Verification items for this drawing (mm, ordinates from the low corner). A direction names the side the tool comes from. Round coordinates to 2 decimals unless told otherwise and drop trailing zeros. Order: outer loops, then holes, each group sorted by start corner. A loop starts at its lowest first (then second) coordinate and runs counter-clockwise, first axis right, second up. Notation, with made-up numbers: M 54,-2 L 67,-2 A22 ccw 67,37 Z; hole C 20.5,-23 d3. An arc over 180 degrees is marked long. One line per item, written item: value. Start each with the question number.
(1) Cross-section at B-B, the plane z = 1.75. Enter the section's corners in (x, y).
(2) Thickness scan on L1, parallel to X at y = 2.25, z = 1.75; L2, parallel to X at y = 3.5, z = 3; L3, parallel to Z at x = 9.25, y = 4.5. Record the ranges inside material, lowest first.
(3) Cross-section at C-C, the plane x = 7.5. Enter the section's corners in (y, z), and give its area (3 significant figures).
(4) Release check for a two-part mould opening along Y. For the marked faces 4, 5 and 6 record: released by +Y, released by -Y, zero draft, split by the parting line, or undercut.
(5) Access from +Z, -Z, +X, -X, +Y, -Y to the whole of each face (thin tool, end or side, straight path). Record for the marked faces 1, 2 and 3.
(6) Cross-section at D-D, the plane z = 3.25. Enter the section's corners in (x, y) (1 decimal).
(7) Cross-section at A-A, the plane y = 3.5. Enter the section's corners in (x, z) (1 decimal).
(8) Depth check by flat-ended pin: pin 1 Ø4 at (x, z) = (11.5, 3.5) entering from -Y; pin 2 Ø1 at (x, z) = (15, 4.5) entering from +Y. Enter the tip coordinate at first touch or a pass-through.
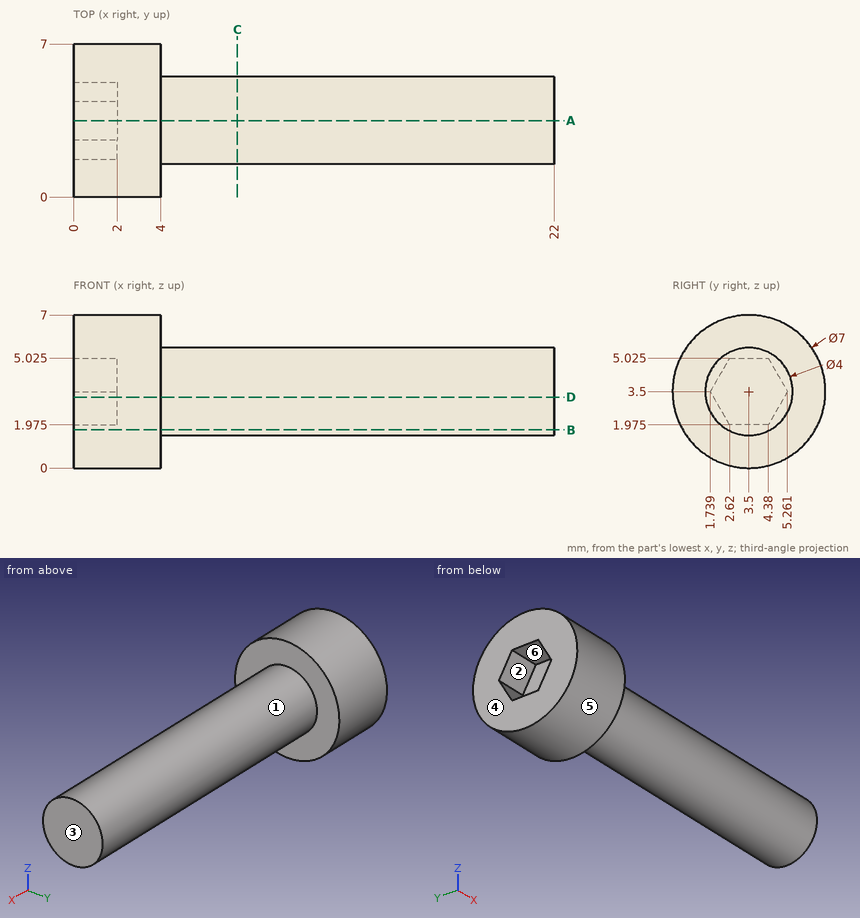
Values found:
1. outline: M 0,0.47 L 4,0.47 L 4,2.53 L 22,2.53 L 22,4.47 L 4,4.47 L 4,6.53 L 0,6.53 Z
2. L1: 0 to 4
2. L2: 2 to 22
2. L3: 1.77 to 5.23
3. outline: C 3.5,3.5 d4
3. area: 12.6 mm^2
4. face 4: zero draft
4. face 5: split by the parting line
4. face 6: undercut
5. face 1: +X
5. face 2: -X
5. face 3: +Z, -Z, +X, +Y, -Y
6. outline: M 0,0 L 4,0 L 4,1.5 L 22,1.5 L 22,5.5 L 4,5.5 L 4,7 L 0,7 L 0,5.1 L 2,5.1 L 2,1.9 L 0,1.9 Z
7. outline: M 0,0 L 4,0 L 4,1.5 L 22,1.5 L 22,5.5 L 4,5.5 L 4,7 L 0,7 L 0,5 L 2,5 L 2,2 L 0,2 Z
8. pin 1: y = 1.5
8. pin 2: y = 5.44
